The listing builds one solid part. Answer for the finished solid, in the listing's coordinates (mm). A direction names the side the tool comes from. Round coordinates to 2 decimals unless told otherwise and drop trailing zeros. Write each loop counter-clockwise with the first axis right and the second up, starting at its lowest first coordinate (ties: lowest second). Pieces come first, ordered by that corner, then holes. Notation, with made-up numbers: (10, 88.5) - (62, 88.5) arc R27 cw to (62, 110.5) - close; hole circle Ø10 at (-22.75, -8). An arc over 180 degrees is marked (long way). Return JSON: item names as keys, results as strings. Group by question number.
Autodesk Inventor part; units mm, degrees
ref_plane "YZ Plane" through (0, 0, 0) normal (1, 0, 0) x (0, 1, 0)
ref_plane "XZ Plane" through (0, 0, 0) normal (0, 1, 0) x (-1, 0, 0)
ref_plane "XY Plane" through (0, 0, 0) normal (0, 0, 1) x (1, 0, 0)
sketch "Sketch1" plane through (0, 0, 0) normal (0, 0, 1) x (1, 0, 0)
  arc A0 (-39.344, -1.4316) -> (39.344, -1.4316) centre (0, 0) ccw
  line L0 (-39.344, -1.4316) -> (-39.3671, -1.4316)
  line L1 (-39.344, -1.4316) -> (-52.044, -1.4316)
  line L2 (39.344, -1.4316) -> (52.044, -1.4316)
  arc A1 (-46.964, -22.4724) -> (46.964, -22.4724) centre (0, 0) ccw
  line L3 (-52.044, -1.4316) -> (-59.664, -1.4316)
  line L4 (52.044, -1.4316) -> (59.664, -1.4316)
  line L5 (39.344, -1.4316) -> (46.964, -1.4316)
  line L6 (46.964, -1.4316) -> (46.964, -22.4724)
  line L7 (-39.344, -1.4316) -> (-45.694, -1.4316)
  line L8 (-39.344, -1.4316) -> (-46.964, -1.4316)
  line L9 (-46.964, -1.4316) -> (-46.964, -22.4724)
  line L10 (-46.964, -7.7816) -> (-59.664, -7.7816)
  line L11 (-59.664, -7.7816) -> (-59.664, -1.4316)
  line L12 (46.964, -7.7816) -> (59.664, -7.7816)
  line L13 (59.664, -7.7816) -> (59.664, -1.4316)
  line L14 (46.964, -42.5386) -> (30.0181, -42.5386)
  line L15 (46.964, -22.4724) -> (46.964, -42.5386)
  line L16 (46.964, -42.5386) -> (-46.964, -42.5386)
  line L17 (-46.964, -42.5386) -> (-46.964, -22.4724)
  line L18 (-46.964, -42.5386) -> (46.964, -42.5386)
  line L19 (46.964, -42.5386) -> (46.964, -52.2316)
  line L20 (46.964, -52.2316) -> (-46.964, -52.2316)
  line L21 (-46.964, -52.2316) -> (-46.964, -42.5386)
  line L22 (-46.964, -22.4724) -> (-32.3263, -22.4724)
  line L23 (32.3263, -22.4724) -> (46.964, -22.4724)
  dimension "d0" = 78.74
  dimension "d1" = 12.7
  dimension "d2" = 12.7
  dimension "d4" = 7.62
  dimension "d5" = 7.62
  dimension "d6" = 7.62
  dimension "d7" = 7.62
  dimension "d8" = 6.35
  dimension "d9" = 6.35
  dimension "d20" = 50.8
extrude "Extrusion1" add sketch "Sketch1" along normal blind 12.7
sketch "Sketch2" plane through (-59.664, -1.4316, 0) normal (0, 1, 0) x (1, 0, 0)
  line L0 (20.32, 0) -> (0, 0)
  line L1 (0, 0) -> (20.32, 0)
  circle A0 centre (7.62, -6.35) radius 4.064
  circle A1 centre (111.7079, -6.35) radius 4.064
  line L2 (99.0079, 0) -> (99.0079, -12.7)
  line L3 (20.32, 0) -> (20.32, -12.7)
  point P0 (59.664, 0)
  dimension "d14" = 12.7
  dimension "d15" = 12.7
  dimension "d16" = 8.128
  dimension "d17" = 8.128
extrude "Extrusion2" cut sketch "Sketch2" against normal blind 25.4
properties part number "MOTOR MOUNT REAL TOP E3O MOTOR"
(1) Find section B-B (y = -6.5). Write down the section's boundary in (x, z), plus the area to 3 significant figures.
(2) Determine the mould class of faces 4 (the cylindrical face through (-48.168, -4.562, 5.129)), 5 (the flat face through (56, -7.782, 8)), 6 (the flat face through (-1, -43, 0)) for opening direction Z: +Z half, -Z half, draft (parallel to the pull), parting line (faces both ways), or undercut.
(3) Consider line 1 (X direction, y = -3.5, z = 8.25); line 2 (X direction, y = -6.5, z = 6.35); line 3 (Y direction, x = -1.5, z = 5.75). Determine where each line is inside the solid, lowest interval first.
(4) Flat-ended cylindrical pins translate along their axes: pin 1 (6.5 mm diameter, centred on y = -36.5, z = 7.5, fed in from -X); pin 2 (4 mm diameter, centred on x = 55.5, z = 3.5, fed in from -Y). Find the tip coordinate at first contact, or state that the pin passes through.
(5) Find section A-A (z = 6.35). Write down the section's boundary in (x, y), plus the area to 3 significant figures.
(6) Find section C-C (x = -50). Write down the section's boundary in (y, z), plus the area to 3 significant figures.
(7) For faces 1 (the flat face through (46.964, -30, 6)), 2 (the flat face through (-46.964, -30, 6)), 3 (the flat face through (-1, -43, 12.7)), determine the directions among +Z, -Z, +X, -X, +Y, -Y from which every point of the face is accessible in a straight line to the end or side of a thin tool.
(8) Find section D-D (y = -14.5). Write down the section's boundary in (x, z).
Check sheet entries:
{
 "1": {"outline": "(-59.66, 0) - (-38.83, 0) - (-38.83, 12.7) - (-59.66, 12.7) - close; (38.83, 0) - (59.66, 0) - (59.66, 12.7) - (38.83, 12.7) - close; hole circle Ø8.13 at (-52.04, 6.35); hole circle Ø8.13 at (52.04, 6.35)", "area": "425 mm^2"},
 "2": {"face 4": "undercut", "face 5": "draft", "face 6": "-Z half"},
 "3": {"line 1": "x = -59.66 to -55.64, -48.45 to -39.21, 39.21 to 48.45, 55.64 to 59.66", "line 2": "x = -59.66 to -56.11, -47.98 to -38.83, 38.83 to 47.98, 56.11 to 59.66", "line 3": "y = -52.23 to -39.34"},
 "4": {"pin 1": "stops at x = -46.96", "pin 2": "stops at y = -7.78"},
 "5": {"outline": "(-59.66, -7.78) - (-56.11, -7.78) - (-56.11, -1.43) - (-59.66, -1.43) - close; (-47.98, -7.78) - (-46.96, -7.78) - (-46.96, -52.23) - (46.96, -52.23) - (46.96, -7.78) - (47.98, -7.78) - (47.98, -1.43) - (39.34, -1.43) arc R39.37 cw to (-39.34, -1.43) - (-47.98, -1.43) - close; (56.11, -7.78) - (59.66, -7.78) - (59.66, -1.43) - (56.11, -1.43) - close", "area": "2,510 mm^2"},
 "6": {"outline": "(-7.78, 0) - (-1.43, 0) - (-1.43, 2.84) - (-7.78, 2.84) - close; (-7.78, 9.86) - (-1.43, 9.86) - (-1.43, 12.7) - (-7.78, 12.7) - close", "area": "36.0 mm^2"},
 "7": {"face 1": "+Z, -Z, +X, -Y", "face 2": "+Z, -Z, -X, -Y", "face 3": "+Z, +X, -X, +Y, -Y"},
 "8": {"outline": "(-46.96, 0) - (-36.6, 0) - (-36.6, 12.7) - (-46.96, 12.7) - close; (36.6, 0) - (46.96, 0) - (46.96, 12.7) - (36.6, 12.7) - close"}
}
